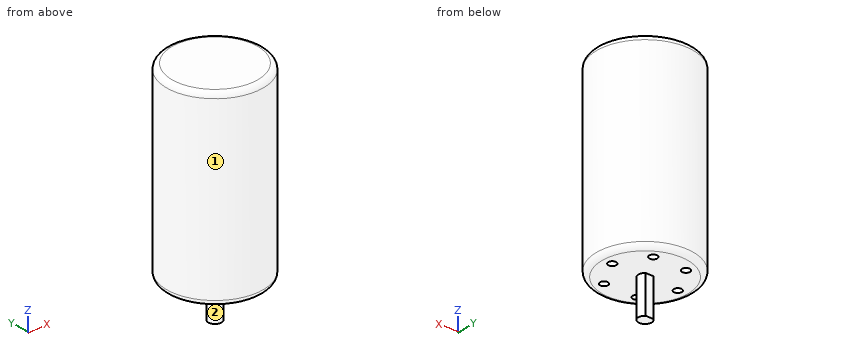
```python
from build123d import *

# Parameters (mm, degrees)
SKETCH1_R           = 18
BOSS_EXTRUDE1_DEPTH = 70
BOSS_EXTRUDE2_DEPTH = 14
FILLET1_R           = 2
SKETCH3_R           = 1.5
CUT_EXTRUDE1_DEPTH  = 10


with BuildPart() as part:
    # Sketch1 → Boss-Extrude1 (new body)
    with BuildSketch(Plane.XY):
        Circle(SKETCH1_R)
    extrude(amount=BOSS_EXTRUDE1_DEPTH)

    # Sketch2 → Boss-Extrude2 (add)
    with BuildSketch(Plane(origin=(0, 0, 0), x_dir=(-1, 0, 0), z_dir=(0, 0, -1))):
        with BuildLine():
            Line((-1.5, 2), (1.5, 2))
            ThreePointArc((1.5, 2), (0, -2.5), (-1.5, 2))
        make_face()
    extrude(amount=BOSS_EXTRUDE2_DEPTH)

    # Fillet1
    fillet1_edges = [part.edges().sort_by_distance(p)[0] for p in [
        (-18, 0, 0),
        (-18, 0, 70),
    ]]
    fillet(fillet1_edges, radius=FILLET1_R)

    # Sketch3 → Cut-Extrude1 (cut)
    with BuildSketch(Plane(origin=(0, 0, 0), x_dir=(-1, 0, 0), z_dir=(0, 0, -1))):
        with Locations((-12.5, 0)):
            Circle(SKETCH3_R)
        with Locations((-6.25, 10.825317547)):
            Circle(SKETCH3_R)
        with Locations((6.25, 10.825317547)):
            Circle(SKETCH3_R)
        with Locations((12.5, 0)):
            Circle(SKETCH3_R)
        with Locations((6.25, -10.825317547)):
            Circle(SKETCH3_R)
        with Locations((-6.25, -10.825317547)):
            Circle(SKETCH3_R)
    extrude(amount=-CUT_EXTRUDE1_DEPTH, mode=Mode.SUBTRACT)


solid = part.part
```
Work out the finished part from the listing and answer in its coordinate system (mm). Face numbers are marked on the shaded views. A direction names the side the tool comes from. Give positions to 0.01 mm unless a question says otherwise; leave off trailing zeros. Loops run counter-clockwise (first coordinate to the right, second up) from the corner with the lowest first, then second, coordinate; pieces in that order, holes last. Notation, with made-up numbers: M -10.5,-10 L 12.5,-10 A29 cw 12.5,10 Z; hole C -4.5,40.25 d3. An arc over 180 degrees is marked long. One line per item, written item: value. Start each with the question number.
1. Find section B-B (y = 0). Give the vertices of the cut face in (x, z).
2. Find the intervals of material crossed by probe 1 along Y at (x, z) = (-6.25, 8.25); probe 2 along Y at (x, z) = (-6, 6); probe 3 along Z at (x, y) = (-6.5, -2), in increasing order.
3. Which of the six approach directions +Z, -Z, +X, -X, +Y, -Y give full straight-line access (tool end or side, diameter ignored) to the marked faces 1 and 2?
4. Find section C-C (z = 39.5). Give the vertices of the cut face in (x, y), and give its area (3 significant figures).
5. Each of these flat-tipped pins is pushed along its axis until it touches: P1, Ø5, axis at x = -12.5, y = 0, coming from the -Z side; P2, Ø0.9, axis at x = 6.5, y = -10.5, coming from the -Z side; P3, Ø12, axis at x = -10.5, z = -2.5, coming from the +Y side. Where does it stop, or does it pass through?
6. Find section A-A (x = 0). Give the vertices of the cut face in (y, z), and give its area (3 significant figures).
Reported:
1. outline: M -18,2 A2 ccw -16,0 L -14,0 L -14,10 L -11,10 L -11,0 L -2.5,0 L -2.5,-14 L 2.5,-14 L 2.5,0 L 11,0 L 11,10 L 14,10 L 14,0 L 16,0 A2 ccw 18,2 L 18,68 A2 ccw 16,70 L -16,70 A2 ccw -18,68 Z
2. probe 1: y = -16.88 to -12.33, -9.33 to 9.33, 12.33 to 16.88
2. probe 2: y = -16.97 to -12.3, -9.35 to 9.35, 12.3 to 16.97
2. probe 3: z = 0 to 70
3. face 1: +Z, -Z
3. face 2: -Z
4. outline: C 0,0 d36
4. area: 1,020 mm²
5. P1: stops at z = 0
5. P2: stops at z = 10
5. P3: stops at y = 16.89
6. outline: M -18,2 A2 ccw -16,0 L -2.5,0 L -2.5,-14 L 2,-14 L 2,0 L 16,0 A2 ccw 18,2 L 18,68 A2 ccw 16,70 L -16,70 A2 ccw -18,68 Z
6. area: 2,580 mm²
